The listing builds one solid part. Answer for the finished solid, in the listing's coordinates (mm). A direction names the side the tool comes from. Give positions to 0.01 mm unless a question says otherwise; leave off trailing zeros. Write each loop counter-clockwise with the first axis right and the second up, starting at its lowest first coordinate (ties: lowest second). Pieces come first, ordered by that corner, then holes. Notation, with made-up numbers: (79, -12.75) - (98, -12.75) arc R24 ccw to (98, 23.25) - close; hole circle Ø7 at (-14, 39). An arc over 180 degrees is marked (long way). Return JSON: item names as keys, results as strings.
Autodesk Inventor part; units mm, degrees
ref_plane "YZ Plane" through (0, 0, 0) normal (1, 0, 0) x (0, 1, 0)
ref_plane "XZ Plane" through (0, 0, 0) normal (0, 1, 0) x (-1, 0, 0)
ref_plane "XY Plane" through (0, 0, 0) normal (0, 0, 1) x (1, 0, 0)
sketch "Sketch1" plane through (0, 0, 0) normal (0, 1, 0) x (-1, 0, 0)
  point P0 (0, 0)
sketch "Sketch2" plane through (0, 0, 0) normal (0, 1, 0) x (-1, 0, 0)
  line L0 (0, 0) -> (0, -90)
  line L1 (0, -90) -> (85, -90)
  line L2 (85, -90) -> (85, 0)
  line L3 (85, 0) -> (0, 0)
  dimension "d0" = 90
  dimension "d1" = 85
extrude "Extrusion1" add sketch "Sketch2" along normal blind 3
sketch "Sketch3" plane through (0, 3, 0) normal (0, 1, 0) x (1, 0, 0)
  line L0 (0, 0) -> (0, 3)
  line L1 (0, 0) -> (0, 90)
  line L2 (0, 3) -> (0, 0)
  line L3 (-85, 90) -> (-85, 0)
  line L4 (0, 90) -> (-85, 90)
  line L5 (-3, 3) -> (-82, 3)
  line L6 (-82, 3) -> (-82, 87)
  line L7 (-82, 87) -> (-3, 87)
  line L8 (-3, 87) -> (-3, 3)
  line L9 (0, 90) -> (-85, 90)
  line L10 (-85, 0) -> (0, 0)
  line L11 (-85, 90) -> (0, 90)
  line L12 (0, 90) -> (0, 0)
  line L13 (0, 0) -> (-85, 0)
  line L14 (-85, 0) -> (-85, 90)
extrude "Extrusion2" add sketch "Sketch3" along normal blind 30
sketch "Sketch7" plane through (-82, 3, -87) normal (0, 0, 1) x (1, 0, 0)
  point P0 (82, -3)
sketch "Sketch8" plane through (0, 33, 0) normal (0, 1, 0) x (1, 0, 0)
  line L0 (-3, 3) -> (-3, 87)
  line L1 (-3, 87) -> (-82, 87)
  line L2 (-82, 87) -> (-82, 3)
  line L3 (-82, 3) -> (-3, 3)
  line L4 (0, 0) -> (0, 90)
  line L5 (0, 90) -> (-85, 90)
  line L6 (-85, 90) -> (-85, 0)
  line L7 (-85, 0) -> (0, 0)
  line L8 (-3, 3) -> (-82, 3)
  line L9 (-82, 3) -> (-82, 87)
  line L10 (-82, 87) -> (-3, 87)
  line L11 (-3, 87) -> (-3, 3)
  line L12 (-85, 90) -> (-85, 0)
  line L13 (0, 0) -> (0, 90)
  line L14 (-85, 90) -> (0, 90)
  line L15 (0, 90) -> (0, 0)
  line L16 (0, 0) -> (-85, 0)
  line L17 (-85, 0) -> (-85, 90)
  line L18 (0, 90) -> (-85, 90)
  line L19 (-85, 91.5) -> (-86.5, 91.5)
  line L20 (0, -1.5) -> (1.5, -1.5)
  line L21 (-86.5, 91.5) -> (1.5, 91.5)
  line L22 (1.5, 91.5) -> (1.5, -1.5)
  line L23 (1.5, -1.5) -> (-86.5, -1.5)
  line L24 (-86.5, -1.5) -> (-86.5, 91.5)
  dimension "d26" = 1.5
  dimension "d27" = 1.5
  dimension "d28" = 1.5
  dimension "d29" = 1.5
extrude "Extrusion5" add sketch "Sketch8" against normal blind 3 contours L21 L22 L20 L23 L24 L19
sketch "Sketch9" plane through (0, 33, 0) normal (0, 1, 0) x (1, 0, 0)
  line L0 (-3, 3) -> (-3, 87)
  line L1 (-3, 87) -> (-82, 87)
  line L2 (-82, 87) -> (-82, 3)
  line L3 (-82, 3) -> (-3, 3)
  line L4 (1.5, 91.5) -> (-86.5, 91.5)
  line L5 (-86.5, 91.5) -> (-86.5, -1.5)
  line L6 (-86.5, -1.5) -> (1.5, -1.5)
  line L7 (1.5, -1.5) -> (1.5, 91.5)
  line L8 (-3, 3) -> (-82, 3)
  line L9 (-82, 3) -> (-82, 87)
  line L10 (-82, 87) -> (-3, 87)
  line L11 (-3, 87) -> (-3, 3)
  line L12 (-82, 3) -> (-82, 87)
  line L13 (-82, 87) -> (-82, 88.5)
  line L14 (-82, 88.5) -> (-83.5, 88.5)
  line L15 (-3, 87) -> (-3, 3)
  line L16 (-3, 3) -> (-1.5, 3)
  line L17 (-1.5, 3) -> (-1.5, 1.5)
  line L18 (-1.5, 1.5) -> (-83.5, 1.5)
  line L19 (-83.5, 1.5) -> (-83.5, 88.5)
  line L20 (-83.5, 88.5) -> (-1.5, 88.5)
  line L21 (-1.5, 88.5) -> (-1.5, 1.5)
  line L22 (-83.5, 88.5) -> (-83.5, 90)
  line L23 (0, 90) -> (-85, 90)
  line L24 (-83.5, 90) -> (-85, 90)
  line L25 (0, 0) -> (0, 90)
  line L26 (0, 0) -> (-85, 0)
  line L27 (-85, 0) -> (-85, 90)
  line L28 (-85, 90) -> (0, 90)
  line L29 (0, 90) -> (0, 0)
  dimension "d33" = 1.5
  dimension "d34" = 1.5
  dimension "d35" = 1.5
  dimension "d36" = 1.5
  dimension "d37" = 1.5
extrude "Extrusion6" cut sketch "Sketch9" against normal blind 0.7 contours L23 L25 L26 L27
sketch "Sketch10" plane through (-82, 3, -87) normal (0, 0, 1) x (1, 0, 0)
  line L0 (0, 30) -> (79, 30)
  line L1 (79, 30) -> (79, 0)
  line L2 (79, 0) -> (0, 0)
  line L3 (0, 0) -> (0, 30)
  line L4 (0, 30) -> (79, 30)
  line L5 (79, 0) -> (0, 0)
  circle A0 centre (39.5, 15) radius 6.4
  point P0 (82, -3)
  dimension "d40" = 12.8
extrude "Extrusion7" cut sketch "Sketch10" against normal blind 3 contours A0
sketch "Sketch11" plane through (-3, 3, -3) normal (0, 0, -1) x (-1, 0, 0)
  line L0 (0, 30) -> (79, 30)
  line L1 (79, 0) -> (0, 0)
  line L2 (0, 0) -> (0, 30)
  line L3 (0, 30) -> (79, 30)
  line L4 (79, 30) -> (79, 0)
  line L5 (79, 30) -> (0, 0)
  line L6 (79, 0) -> (0, 0)
  line L7 (0, 30) -> (79, 0)
  circle A0 centre (39.5, 15) radius 6.5
  point P0 (-3, -3)
  dimension "d43" = 13
extrude "Extrusion8" cut sketch "Sketch11" against normal blind 3 contours A0 L5 L7 | L7 L5 A0 | A0 L7 L5 | L5 L7 A0
sketch "Sketch12" plane through (0, 3, 0) normal (0, 1, 0) x (1, 0, 0)
  line L0 (-3, 3) -> (-3, 87)
  line L1 (-3, 87) -> (-82, 87)
  line L2 (-82, 87) -> (-82, 3)
  line L3 (-82, 3) -> (-3, 3)
  line L4 (-3, 87) -> (-3, 3)
  line L5 (-3, 3) -> (-82, 3)
  line L6 (-82, 87) -> (-3, 87)
  line L7 (-71.9395, 76.9395) -> (-13.0605, 13.0605) construction
  line L8 (-13.0605, 76.9395) -> (-71.9395, 13.0605) construction
  circle A0 centre (-13.0605, 13.0605) radius 5
  circle A1 centre (-13.0605, 76.9395) radius 5
  circle A2 centre (-71.9395, 76.9395) radius 5
  line L9 (-66.9395, 13.0605) -> (-62.9395, 13.0605) construction
  circle A3 centre (-71.9395, 13.0605) radius 5
  point P0 (0, 0)
  point P1 (-42.5, 45)
  dimension "d60" = 10
  dimension "d61" = 10
  dimension "d62" = 10
  dimension "d65" = 10
extrude "Extrusion10" add sketch "Sketch12" along normal blind 4 contours A0 | A1 | A2 | A3
sketch "Sketch14" plane through (-71.9395, 7, -13.0605) normal (0, 1, 0) x (1, 0, 0)
  circle A0 centre (0, 0) radius 5
  circle A1 centre (0, 63.879) radius 5
  circle A2 centre (58.879, 0) radius 5
  circle A3 centre (58.879, 63.879) radius 5
  circle A4 centre (0, 0) radius 5
  circle A5 centre (0, 0) radius 5
  circle A6 centre (0, 63.879) radius 5
  circle A7 centre (0, 63.879) radius 5
  circle A8 centre (58.879, 63.879) radius 5
  circle A9 centre (58.879, 0) radius 5
  line L0 (0, 0) -> (-3.5355, 3.5355)
  line L1 (0, 0) -> (5, 0) construction
  line L2 (-3.5355, 3.5355) -> (3.5355, -3.5355)
  line L3 (0, 63.879) -> (-3.5355, 60.3435)
  line L4 (-3.5355, 60.3435) -> (3.5355, 67.4145)
  line L5 (58.879, 63.879) -> (55.3435, 67.4145)
  circle A10 centre (58.879, 63.879) radius 5
  line L6 (55.3435, 67.4145) -> (62.4145, 60.3435)
  line L7 (58.879, 0) -> (55.3435, -3.5355)
  circle A11 centre (58.879, 0) radius 5
  line L8 (55.3435, -3.5355) -> (62.4145, 3.5355)
  point P0 (71.9395, -13.0605)
  point P1 (62.4145, 3.5355)
  point P2 (3.5355, 67.4145)
  point P3 (-3.5355, 60.3435)
  point P4 (3.5355, -3.5355)
  point P5 (-3.5355, 3.5355)
  dimension "d68" = 135
extrude "Extrusion11" cut sketch "Sketch14" against normal blind 4 contours A0 L2 L0 | A1 L3 L4 | L8 L7 A2 | L5 L6 A3 picked at (2.7524, 1.8391) picked at (3.1056, 62.7333) picked at (57.1671, 2.8318) picked at (55.576, 63.6792)
sketch "Sketch15" plane through (0, 7, 0) normal (0, 1, 0) x (1, 0, 0)
  line L0 (-68.404, 9.525) -> (-75.475, 16.596)
  arc A0 (-75.475, 16.596) -> (-68.404, 9.525) centre (-71.9395, 13.0605) ccw
  line L1 (-75.475, 73.404) -> (-68.404, 80.475)
  arc A1 (-68.404, 80.475) -> (-75.475, 73.404) centre (-71.9395, 76.9395) ccw
  line L2 (-16.596, 80.475) -> (-9.525, 73.404)
  arc A2 (-9.525, 73.404) -> (-16.596, 80.475) centre (-13.0605, 76.9395) ccw
  line L3 (-9.525, 16.596) -> (-16.596, 9.525)
  arc A3 (-16.596, 9.525) -> (-9.525, 16.596) centre (-13.0605, 13.0605) ccw
  circle A4 centre (-71.9395, 13.0605) radius 3.5
  circle A5 centre (-71.9395, 76.9395) radius 3.5
  circle A6 centre (-13.0605, 76.9395) radius 3.5
  circle A7 centre (-13.0605, 13.0605) radius 3.5
  point P0 (0, 0)
  dimension "d71" = 7
  dimension "d72" = 7
  dimension "d73" = 7
  dimension "d74" = 7
extrude "Extrusion12" cut sketch "Sketch15" against normal blind 4 contours A4 L0 | L0 A4 | A5 L1 | L1 A5 | A6 L2 | L2 A6 | A7 L3 | L3 A7
sketch "Sketch16" plane through (0, 7, 0) normal (0, 1, 0) x (1, 0, 0)
  arc A0 (-74.4144, 15.5354) -> (-69.4646, 10.5856) centre (-71.9395, 13.0605) ccw
  line L0 (-74.4144, 15.5354) -> (-75.475, 16.596)
  arc A1 (-75.475, 16.596) -> (-68.404, 9.525) centre (-71.9395, 13.0605) ccw
  line L1 (-68.404, 9.525) -> (-69.4646, 10.5856)
  arc A2 (-15.5354, 10.5856) -> (-10.5856, 15.5354) centre (-13.0605, 13.0605) ccw
  line L2 (-15.5354, 10.5856) -> (-16.596, 9.525)
  arc A3 (-16.596, 9.525) -> (-9.525, 16.596) centre (-13.0605, 13.0605) ccw
  line L3 (-9.525, 16.596) -> (-10.5856, 15.5354)
  arc A4 (-10.5856, 74.4646) -> (-15.5354, 79.4144) centre (-13.0605, 76.9395) ccw
  line L4 (-10.5856, 74.4646) -> (-9.525, 73.404)
  arc A5 (-9.525, 73.404) -> (-16.596, 80.475) centre (-13.0605, 76.9395) ccw
  line L5 (-16.596, 80.475) -> (-15.5354, 79.4144)
  arc A6 (-69.4646, 79.4144) -> (-74.4144, 74.4646) centre (-71.9395, 76.9395) ccw
  line L6 (-69.4646, 79.4144) -> (-68.404, 80.475)
  arc A7 (-68.404, 80.475) -> (-75.475, 73.404) centre (-71.9395, 76.9395) ccw
  line L7 (-75.475, 73.404) -> (-74.4144, 74.4646)
  circle A8 centre (-71.9395, 13.0605) radius 5
  arc A9 (-68.404, 80.475) -> (-75.475, 73.404) centre (-71.9395, 76.9395) ccw
  circle A10 centre (-71.9395, 76.9395) radius 5
  circle A11 centre (-13.0605, 76.9395) radius 5
  circle A12 centre (-13.0605, 13.0605) radius 5
  point P0 (0, 0)
  point P1 (-75.475, 73.404)
  point P2 (-16.596, 80.475)
  point P3 (-68.404, 9.525)
  point P4 (-9.525, 16.596)
extrude "Extrusion13" add sketch "Sketch16" along normal blind 4
sketch "Sketch17" plane through (-13.0605, 11, -76.9395) normal (0, 1, 0) x (1, 0, 0)
  circle A0 centre (0, 0) radius 5
  circle A1 centre (0, -63.879) radius 5
  circle A2 centre (-58.879, 0) radius 5
  circle A3 centre (-58.879, -63.879) radius 5
  circle A4 centre (0, 0) radius 1.75
  arc A5 (3.5355, -60.3435) -> (-3.5355, -67.4145) centre (0, -63.879) ccw
  circle A6 centre (0, -63.879) radius 1.75
  circle A7 centre (-58.879, -63.879) radius 1.75
  circle A8 centre (-58.879, 0) radius 5
  circle A9 centre (-58.879, 0) radius 1.75
  point P0 (13.0605, -76.9395)
  dimension "d79" = 3.5
  dimension "d80" = 3.5
  dimension "d81" = 3.5
  dimension "d82" = 3.5
extrude "Extrusion14" cut sketch "Sketch17" against normal blind 4 contours A4 | A6 | A7 | A9
sketch "Sketch18" plane through (1.5, 33, -91.5) normal (0, 0, -1) x (-1, 0, 0)
  point P0 (1.5, -33)
sketch "Sketch20" plane through (0, 33, 0) normal (0, 1, 0) x (1, 0, 0)
  line L0 (1.5, 91.5) -> (1.5, -1.5)
  line L1 (1.5, -1.5) -> (5.0355, -5.0355)
  line L2 (1.5, -1.5) -> (6.5, -1.5) construction
  circle A0 centre (5.0355, -5.0355) radius 5
  line L3 (5.0355, -5.0355) -> (8.5711, -1.5)
  line L4 (8.5711, -1.5) -> (1.5, -8.5711)
  line L5 (1.5, -8.5711) -> (-5.5711, -1.5)
  line L6 (1.5, -1.5) -> (-86.5, -1.5)
  line L7 (8.5711, -1.5) -> (1.5, 5.5711)
  line L8 (-86.5, 91.5) -> (-86.5, -1.5)
  line L9 (-86.5, -1.5) -> (-90.0355, -5.0355)
  line L10 (-86.5, -1.5) -> (-81.5, -1.5) construction
  circle A1 centre (-90.0355, -5.0355) radius 5
  line L11 (-90.0355, -5.0355) -> (-86.5, -8.5711)
  line L12 (-86.5, -8.5711) -> (-93.5711, -1.5)
  line L13 (-93.5711, -1.5) -> (-86.5, 5.5711)
  line L14 (-86.5, -8.5711) -> (-79.4289, -1.5)
  line L15 (-86.5, 91.5) -> (-90.0355, 95.0355)
  line L16 (-86.5, 91.5) -> (-81.5, 91.5) construction
  circle A2 centre (-90.0355, 95.0355) radius 5
  line L17 (-90.0355, 95.0355) -> (-93.5711, 91.5)
  line L18 (-93.5711, 91.5) -> (-86.5, 98.5711)
  line L19 (-93.5711, 91.5) -> (-86.5, 84.4289)
  line L20 (-86.5, 98.5711) -> (-79.4289, 91.5)
  line L21 (-86.5, 91.5) -> (1.5, 91.5)
  line L22 (1.5, 91.5) -> (5.0355, 95.0355)
  line L23 (1.5, 91.5) -> (6.5, 91.5) construction
  circle A3 centre (5.0355, 95.0355) radius 5
  line L24 (5.0355, 95.0355) -> (8.5711, 91.5)
  line L25 (8.5711, 91.5) -> (1.5, 98.5711)
  line L26 (1.5, 98.5711) -> (-5.5711, 91.5)
  line L27 (8.5711, 91.5) -> (1.5, 84.4289)
  point P0 (0, 0)
  dimension "d85" = 5
  dimension "d86" = 45
  dimension "d87" = 5
  dimension "d88" = 135
  dimension "d89" = 5
  dimension "d90" = 135
  dimension "d91" = 5
  dimension "d92" = 45
extrude "Extrusion15" add sketch "Sketch20" against normal blind 3 contours A3 L27 L0 | A3 L25 L22 | L21 L26 A3 | L22 L24 A3 | L25 A3 L24 | L7 A0 L0 | L21 A2 L20 | A0 L3 L1 | L1 L4 A0 | A0 L5 L6 | A0 L4 L3 | L18 L17 A2 | A2 L15 L18 | A2 L17 L15 | L8 L19 A2 | L14 A1 L6 | L8 A1 L13 | A1 L11 L9 | L9 L12 A1 | A1 L12 L11
sketch "Sketch21" plane through (0, 33, 0) normal (0, 1, 0) x (1, 0, 0)
  line L0 (-5.5711, 91.5) -> (-79.4289, 91.5)
  line L1 (-79.4289, 91.5) -> (-86.5, 98.5711)
  arc A0 (-86.5, 98.5711) -> (-93.5711, 91.5) centre (-90.0355, 95.0355) ccw
  line L2 (-93.5711, 91.5) -> (-86.5, 84.4289)
  line L3 (-86.5, 84.4289) -> (-86.5, 5.5711)
  line L4 (-86.5, 5.5711) -> (-93.5711, -1.5)
  arc A1 (-93.5711, -1.5) -> (-86.5, -8.5711) centre (-90.0355, -5.0355) ccw
  line L5 (-86.5, -8.5711) -> (-79.4289, -1.5)
  line L6 (-79.4289, -1.5) -> (-5.5711, -1.5)
  line L7 (-5.5711, -1.5) -> (1.5, -8.5711)
  arc A2 (1.5, -8.5711) -> (8.5711, -1.5) centre (5.0355, -5.0355) ccw
  line L8 (8.5711, -1.5) -> (1.5, 5.5711)
  line L9 (1.5, 5.5711) -> (1.5, 84.4289)
  line L10 (1.5, 84.4289) -> (8.5711, 91.5)
  arc A3 (8.5711, 91.5) -> (1.5, 98.5711) centre (5.0355, 95.0355) ccw
  line L11 (1.5, 98.5711) -> (-5.5711, 91.5)
  line L12 (0, 0) -> (-85, 0)
  line L13 (-85, 0) -> (-85, 90)
  line L14 (-85, 90) -> (0, 90)
  line L15 (0, 90) -> (0, 0)
  circle A4 centre (5.0355, -5.0355) radius 1.75
  circle A5 centre (5.0355, 95.0355) radius 1.75
  circle A6 centre (-90.0355, 95.0355) radius 1.75
  circle A7 centre (-90.0355, -5.0355) radius 1.75
  dimension "d95" = 3.5
  dimension "d96" = 3.5
  dimension "d97" = 3.5
  dimension "d98" = 3.5
extrude "Extrusion16" cut sketch "Sketch21" against normal blind 3 contours A4 | A5 | A6 | A7
properties part number "Base inferior" material "Steel, Mild, Welded"
Item 1: For faces 1 (the face through (-43, 32, -91.5)), 2 (the face through (-10.53, 5.03, -79.36)), 3 (the face through (-93.65, 31.52, 8.49)), 4 (the face through (-1.986, 31.521, 5.085)), 5 (the face through (-72, 11, -11)), determine the directions among +Z, -Z, +X, -X, +Y, -Y from which every point of the face is accessible in a straight line to the end or side of a thin tool.
Answer below:
{"face 1": "-Z, +Y, -Y", "face 2": "none", "face 3": "+Y, -Y", "face 4": "+Z, +Y, -Y", "face 5": "+Y"}
Item 2: A cutting plane is placed at D-D on y = 18. Determine the outline of the cut face in (x, z).
Answer below:
{"outline": "(-85, -90) - (-48.9, -90) - (-48.9, -87) - (-82, -87) - (-82, -3) - (-49, -3) - (-49, 0) - (-85, 0) - close; (-36.1, -90) - (0, -90) - (0, 0) - (-36, 0) - (-36, -3) - (-3, -3) - (-3, -87) - (-36.1, -87) - close"}
Item 3: The mould has two halves that part along Z. Classify faces 6 (the face through (-42, 11, -90)), 7 (the face through (-70, 7, -14)), 8 (the face through (-43, 32, 1.5)), 9 (the face through (-3, 18, -46)): +Z half, -Z half, draft (parallel to the pull), parting line (faces both ways), or undercut.
Answer below:
{"face 6": "-Z half", "face 7": "undercut", "face 8": "+Z half", "face 9": "undercut"}
Item 4: A cutting plane is placed at B-B on x = -42.5. Determine the outline of the cut face in (y, z).
Answer below:
{"outline": "(0, -90) - (11.6, -90) - (11.6, -87) - (3, -87) - (3, -3) - (11.5, -3) - (11.5, 0) - (0, 0) - close; (24.4, -90) - (30, -90) - (30, -91.5) - (33, -91.5) - (33, -90) - (32.3, -90) - (32.3, -88.5) - (33, -88.5) - (33, -87) - (24.4, -87) - close; (24.5, -3) - (33, -3) - (33, -1.5) - (32.3, -1.5) - (32.3, 0) - (33, 0) - (33, 1.5) - (30, 1.5) - (30, 0) - (24.5, 0) - close"}
Item 5: Flat-ended cylindrical pins translate along their axes: P1, Ø2, axis at x = -90.04, z = 5.04, coming from the +Y side; P2, Ø9, axis at x = -33.5, y = 11, coming from the +Z side; P3, Ø5, axis at y = 28, z = -20.5, coming from the -X side; P4, Ø3, axis at y = 9, z = -11, coming from the -X side. Find the tip coordinate at first contact, or state that the pin passes through.
Answer below:
{"P1": "passes through", "P2": "stops at z = 0", "P3": "stops at x = -86.5", "P4": "stops at x = -85"}
Item 6: A cutting plane is placed at A-A on y = 5.5. Determine the outline of the cut face in (x, z) (1 decimal).
Answer below:
{"outline": "(-85, -90) - (0, -90) - (0, 0) - (-85, 0) - close; (-75.5, -73.4) arc R5 ccw to (-68.4, -80.5) - (-69.5, -79.4) arc R3.5 cw to (-74.4, -74.5) - close; (-75.5, -16.6) - (-74.4, -15.5) arc R3.5 cw to (-69.5, -10.6) - (-68.4, -9.5) arc R5 ccw to start; (-16.6, -80.5) arc R5 ccw to (-9.5, -73.4) - (-10.6, -74.5) arc R3.5 cw to (-15.5, -79.4) - close; (-16.6, -9.5) - (-15.5, -10.6) arc R3.5 cw to (-10.6, -15.5) - (-9.5, -16.6) arc R5 ccw to start; hole (-82, -87) - (-3, -87) - (-3, -3) - (-82, -3) - close"}
Item 7: Consider L1, parallel to X at y = 27, z = -22; L2, parallel to Z at x = -16, y = 14.5; L3, parallel to Y at x = -42.5, z = -87.7. Determine where each line is inside the solid, lowest interval first.
Answer below:
{"L1": "x = -85 to -82, -3 to 0", "L2": "z = -90 to -87, -3 to 0", "L3": "y = 0 to 11.6, 24.4 to 33"}
Item 8: A cutting plane is placed at C-C on z = -30. Determine the outline of the cut face in (x, y).
Answer below:
{"outline": "(-86.5, 30) - (-85, 30) - (-85, 0) - (0, 0) - (0, 30) - (1.5, 30) - (1.5, 33) - (0, 33) - (0, 32.3) - (-1.5, 32.3) - (-1.5, 33) - (-3, 33) - (-3, 3) - (-82, 3) - (-82, 33) - (-83.5, 33) - (-83.5, 32.3) - (-85, 32.3) - (-85, 33) - (-86.5, 33) - close"}
